from build123d import *

# Parameters (mm, degrees)
BOSS_EXTRUDE1_DEPTH             = 138
SKETCH10_R                      = 150
BOSS_EXTRUDE6_DEPTH             = 220
BOSS_EXTRUDE6_DIRECTION_2_REACH = 314.006
SPLIT3_DEPTH                    = 76
FILLET2_R                       = 200
BOSS_EXTRUDE7_DEPTH             = 109.159437572


with BuildPart() as part:
    # Sketch1 → Boss-Extrude1 (new body)
    with BuildSketch(Plane(origin=(0, 0, 0), x_dir=(1, 0, 0), z_dir=(0, 1, 0))):
        with BuildLine():
            Line((8.485281374, 8.485281374), (150, 150))
            Line((150, 150), (278.911017507, 150))
            Line((278.911017507, 150), (278.911017507, -150))
            Line((278.911017507, -150), (150, -150))
            Line((150, -150), (8.485281374, -8.485281374))
            ThreePointArc((8.485281374, -8.485281374), (12, 0), (8.485281374, 8.485281374))
        make_face()
    extrude(amount=BOSS_EXTRUDE1_DEPTH)

    # Split1
    split(bisect_by=Plane(origin=(0, 0, 0), x_dir=(-0.8660254037844416, -0.49999999999999495, 0), z_dir=(0.49999999999999495, -0.8660254037844416, 0)), keep=Keep.BOTTOM)

    # Sketch10 → Boss-Extrude6 (add)
    with BuildSketch(Plane(origin=(0, 138, 0), x_dir=(1, 0, 0), z_dir=(0, 1, 0))):
        with Locations(Location((239.023011445, 0, 0), (0, 0, 270))):
            Circle(SKETCH10_R)
    extrude(amount=BOSS_EXTRUDE6_DEPTH)

    # Boss-Extrude6 direction 2: up to this face of the body (flat: up to its plane)
    boss_extrude6_direction_2_end = Plane(part.part.faces().sort_by_distance((151.627791868, 87.542346451, 0))[0])
    # Sketch10 → Boss-Extrude6 direction 2 (add, up to the picked face)
    with BuildSketch(Plane(origin=(0, 138, 0), x_dir=(1, 0, 0), z_dir=(0, 1, 0)), mode=Mode.PRIVATE) as boss_extrude6_direction_2_sk1:
        with Locations(Location((239.023011445, 0, 0), (0, 0, 270))):
            Circle(SKETCH10_R)
    boss_extrude6_direction_2_tool1 = split(extrude(boss_extrude6_direction_2_sk1.sketch, amount=-BOSS_EXTRUDE6_DIRECTION_2_REACH, mode=Mode.PRIVATE), bisect_by=boss_extrude6_direction_2_end, keep=Keep.BOTH, mode=Mode.PRIVATE)
    add(boss_extrude6_direction_2_tool1.solids().sort_by(Axis((239.023011, 138, 0), (0, -1, 0)))[0])

    # Split3: read off the stored shape, not the designer's step
    # Split3 outline → Split3 (cut)
    with BuildSketch(Plane(origin=(0, 0, 0), x_dir=(0.8660254037844416, 0.4999999999999948, 0), z_dir=(0.4999999999999948, -0.8660254037844417, 0))):
        with BuildLine():
            Line((173.205080757, -150), (276, -150))
            add(Edge.make_bspline(
                [(276, -150), (449.205080757, -150), (449.205080757, 0), (449.205080757, 150), (276, 150)],
                knots=[4.71238898, 4.71238898, 4.71238898, 6.283185307, 6.283185307, 7.853981634, 7.853981634, 7.853981634], degree=2, weights=[1, 0.707106781, 1, 0.707106781, 1]))
            Line((276, 150), (173.205080757, 150))
            Line((173.205080757, 150), (9.797958971, 8.485281374))
            add(Edge.make_bspline(
                [(9.797958971, -8.485281374), (19.595917942, 0), (9.797958971, 8.485281374)],
                knots=[2.35619449, 2.35619449, 2.35619449, 3.926990817, 3.926990817, 3.926990817], degree=2, weights=[1, 0.707106781, 1]))
            Line((9.797958971, -8.485281374), (173.205080757, -150))
        make_face()
    extrude(amount=SPLIT3_DEPTH, mode=Mode.SUBTRACT)

    # Fillet2
    fillet2_edges = [part.edges().sort_by_distance(p)[0] for p in [
        (150, 112.301270189, -150),
        (150, 112.301270189, 150),
    ]]
    fillet(fillet2_edges, radius=FILLET2_R)

    # Sketch12 → Boss-Extrude7 (add, along a direction that is not the sketch's normal)
    with BuildSketch(Plane(origin=(0, 0, 0), x_dir=(0.8660254037844417, 0.49999999999999495, 0), z_dir=(0.49999999999999495, -0.8660254037844417, 0))):
        with BuildLine():
            Line((9.797958971, -8.485281374), (105.564289267, -91.421356237))
            add(Edge.make_bspline(
                [(105.564289267, -91.421356237), (173.205080757, -150), (268.863605452, -150)],
                knots=[0.785398163, 0.785398163, 0.785398163, 1.570796327, 1.570796327, 1.570796327], degree=2, weights=[1, 0.923879533, 1]))
            Line((268.863605452, -150), (276, -150))
            add(Edge.make_bspline(
                [(276, -150), (449.205080757, -150), (449.205080757, 0), (449.205080757, 150), (276, 150)],
                knots=[4.71238898, 4.71238898, 4.71238898, 6.283185307, 6.283185307, 7.853981634, 7.853981634, 7.853981634], degree=2, weights=[1, 0.707106781, 1, 0.707106781, 1]))
            Line((276, 150), (268.863605452, 150))
            add(Edge.make_bspline(
                [(268.863605452, 150), (173.205080757, 150), (105.564289267, 91.421356237)],
                knots=[4.71238898, 4.71238898, 4.71238898, 5.497787144, 5.497787144, 5.497787144], degree=2, weights=[1, 0.923879533, 1]))
            Line((105.564289267, 91.421356237), (9.797958971, 8.485281374))
            add(Edge.make_bspline(
                [(9.797958971, -8.485281374), (19.595917942, 0), (9.797958971, 8.485281374)],
                knots=[2.35619449, 2.35619449, 2.35619449, 3.926990817, 3.926990817, 3.926990817], degree=2, weights=[1, 0.707106781, 1]))
        make_face()
    extrude(amount=-BOSS_EXTRUDE7_DEPTH, dir=(0, -1, 0))


solid = part.part
Build history of the part. All positions in model axes, mm. A direction names the side the tool comes from. Coordinates: 2 decimals unless noted, no trailing zeros. Order: outer loops, then holes, each group sorted by start corner. A loop starts at its lowest first (then second) coordinate and runs counter-clockwise, first axis right, second up. Notation, with made-up numbers: (-19.5, 22.5) - (26.5, 22.5) arc R29 cw to (26.5, 57.5) - close; hole circle Ø3 at (-13, 4.25). An arc over 180 degrees is marked (long way). Write item = value, one per line. Start each with the question number.
1) Saw through at A-A on z = 0. Write the cut outline in (x, y), then the cut area to 3 significant figures.
2) Two-plate mould, pull along Z, no slides. Class faces 1 (the face through (12, 71, 0)), 2 (the face through (141.47, 105.456, 127.907)), 3 (the face through (88.026, 159.981, 0.7)), 4 (the face through (139.52, 105.46, -126.89)): pulls with the +Z half, pulls with the -Z half, needs draft (parallel to the pull), parting line crosses it, or undercut.
3) Saw through at C-C on z = 57. Write the cut outline in (x, y), then the cut area to 3 significant figures.
4) 3-axis set-ups, long thin cutter, end or side, ignore diameter. For faces 5 (the face through (92.59, 270.9, -32.52)), 6 (the face through (201.42, 116.29, -2.1)), 7 (the face through (34, 138, -1)): which of +Z, -Z, +X, -X, +Y, -Y reach the whole face in a straight line?
5) Flat gauge pins, fed straight in: pin 1 Ø10 at (y, z) = (186.5, -75.5) entering from +X; pin 2 Ø1 at (x, y) = (87, 60) entering from -Z; pin 3 Ø10 at (y, z) = (267, -48) entering from +X. Where does each tip first touch, or does it go through?
6) Saw through at D-D on y = 33.5. Write the cut outline in (x, z).
7) Saw through at B-B on x = 58. Write the cut outline in (y, z).
8) Wall check: line 1 along Y through (x, z) = (318, 42.5); line 2 along Z through (x, y) = (212, 260); line 3 along X through (y, z) = (155.5, -131.5). Give the ranges that are in metal, low to high. Write a range as from..to.
From the geometry:
q1.outline = (12, 6.93) - (389.02, 224.6) - (389.02, 358) - (89.02, 358) - (89.02, 160.56) - (49.95, 138) - (12, 138) - close
q1.area = 74,800 mm^2
q2.face_1 = undercut
q2.face_2 = pulls with the +Z half
q2.face_3 = needs draft
q2.face_4 = pulls with the -Z half
q3.outline = (57, 32.91) - (377.77, 218.11) - (377.77, 358) - (100.28, 358) - (100.28, 167.05) - (57, 142.07) - close
q3.area = 65,800 mm^2
q4.face_5 = +Y
q4.face_6 = +Z, -Z, +X, -Y
q4.face_7 = +Z, -Z, -X, +Y
q5.pin_1 = 331.69
q5.pin_2 = -87.5
q5.pin_3 = 382.73
q6.outline = (8.49, -8.49) - (58.02, -58.02) - (58.02, 58.02) - (8.49, 8.49) arc R12 cw to start
q7.outline = (33.49, -58) - (142.65, -58) - (142.65, 58) - (33.49, 58) - close
q8.line_1 = 183.6..358
q8.line_2 = -147.55..147.55
q8.line_3 = 148.83..269.33
